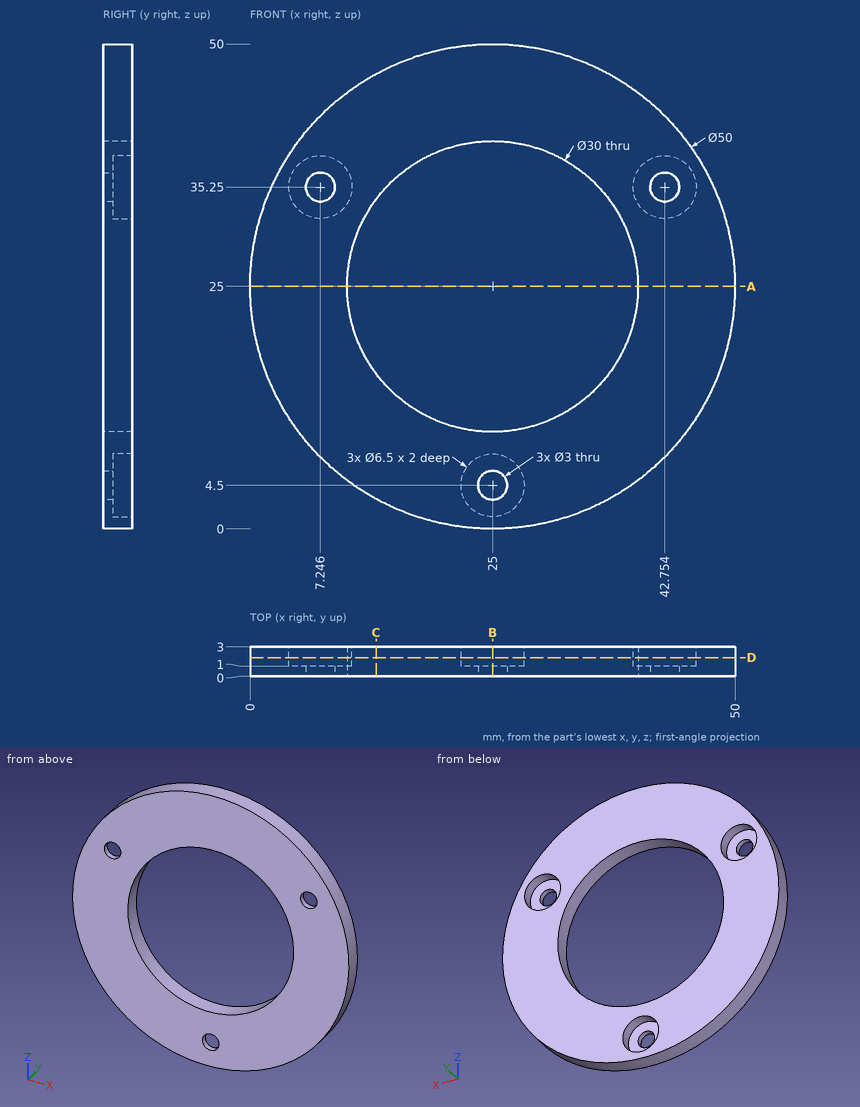
Design review of the part shown in the three views and the two pictorial views. Dimensions are in mm from the part's minimum x, y and z. Round coordinates to 2 decimals unless told otherwise and drop trailing zeros. Write each loop counter-clockwise with the first axis right and the second up, starting at its lowest first coordinate (ties: lowest second). Pieces come first, ordered by that corner, then holes.
Item 1: Clearance check with flat-ended pins moving along their axes: pin 1 Ø4 at (x, z) = (7.25, 35.25) entering from -Y; pin 2 Ø5 at (x, z) = (7.25, 35.25) entering from +Y; pin 3 Ø1 at (x, y) = (5.5, 0.5) entering from +Z; pin 4 Ø1 at (y, z) = (1.5, 26) entering from -X (1 decimal). State where each tip first meets the part, or that it passes through.
Item 2: We need section D-D on y = 1.9. Write out the cut boundary in (x, z).
Item 3: We need section B-B on x = 25. Write out the cut boundary in (y, z), and give its area (3 significant figures).
Item 4: For probe 1 along X at (y, z) = (2.1, 37) (1 decimal); probe 2 along Z at (x, y) = (21, 0.7); probe 3 along X at (y, z) = (1.9, 25), list the stretches that pass through material, from the lowest coordinate up.
Item 5: We need section A-A on z = 25. Write out the cut boundary in (x, y).
Item 6: We need section C-C on x = 13. Write out the cut boundary in (y, z).
Returned:
1. pin 1: stops at y = 0
1. pin 2: stops at y = 1
1. pin 3: stops at z = 41.25
1. pin 4: stops at x = 0
2. outline: circle Ø50 at (25, 25); hole circle Ø6.5 at (7.25, 35.25); hole circle Ø30 at (25, 25); hole circle Ø6.5 at (25, 4.5); hole circle Ø6.5 at (42.75, 35.25)
3. outline: (0, 0) - (3, 0) - (3, 1.25) - (1, 1.25) - (1, 3) - (0, 3) - close; (0, 6) - (1, 6) - (1, 7.75) - (3, 7.75) - (3, 10) - (0, 10) - close; (0, 40) - (3, 40) - (3, 50) - (0, 50) - close
3. area: 44.0 mm2
4. probe 1: x = 3.1 to 4.5, 10 to 16, 34 to 40, 45.5 to 46.9
4. probe 2: z = 0.32 to 10.54, 39.46 to 49.68
4. probe 3: x = 0 to 10, 40 to 50
5. outline: (0, 0) - (10, 0) - (10, 3) - (0, 3) - close; (40, 0) - (50, 0) - (50, 3) - (40, 3) - close
6. outline: (0, 3.07) - (3, 3.07) - (3, 16) - (0, 16) - close; (0, 34) - (3, 34) - (3, 46.93) - (0, 46.93) - close
